Can you work these out from the model? Positions are in its coordinate system, mm. A direction names the side the tool comes from. Give positions to 0.01 mm unless a question says otherwise; leave off trailing zeros. Order: outer loops, then holes, each group sorted by start corner. A loop starts at its lowest first (then second) coordinate and runs counter-clockwise, first axis right, second up. Notation, with made-up numbers: (-12.5, 42.25) - (-4.5, 42.25) arc R23 cw to (-4.5, 62.25) - close; hole circle Ø9 at (43.25, -5.5). An arc over 180 degrees is marked (long way). Answer as a JSON object with one key per item and string values.
```python
from build123d import *

# Parameters (mm, degrees)
SKETCH1_W           = 27.99800038
SKETCH1_H           = 2
BOSS_EXTRUDE1_DEPTH = 10
CUT_EXTRUDE1_DEPTH  = 32
SKETCH4_W           = 27.99800038
SKETCH4_H           = 2
BOSS_EXTRUDE2_DEPTH = 22.81231465
SKETCH5_W           = 4.9
SKETCH5_H           = 2
BOSS_EXTRUDE3_DEPTH = 27.99800038


with BuildPart() as part:
    # Sketch1 → Boss-Extrude1 (new body)
    with BuildSketch(Plane(origin=(0, 0, 0), x_dir=(1, 0, 0), z_dir=(0, 1, 0))):
        with Locations((13.99900019, 1)):
            Rectangle(SKETCH1_W, SKETCH1_H)
    extrude(amount=BOSS_EXTRUDE1_DEPTH)

    # Sketch3 → Cut-Extrude1 (cut)
    with BuildSketch(Plane(origin=(27.99800038, 0, 0), x_dir=(0, 0, -1), z_dir=(1, 0, 0))):
        Polygon((1, 8.25), (2, 8.25), (2, 0), (0, 0), (0, 1), align=None)
    extrude(amount=-CUT_EXTRUDE1_DEPTH, mode=Mode.SUBTRACT)

    # Sketch4 → Boss-Extrude2 (add)
    with BuildSketch(Plane(origin=(0, 10, 0), x_dir=(1, 0, 0), z_dir=(0, 1, 0))):
        with Locations((13.99900019, 1)):
            Rectangle(SKETCH4_W, SKETCH4_H)
    extrude(amount=BOSS_EXTRUDE2_DEPTH)

    # Sketch5 → Boss-Extrude3 (add)
    with BuildSketch(Plane(origin=(27.99800038, 0, 0), x_dir=(0, 0, -1), z_dir=(1, 0, 0))):
        with Locations((2.45, 31.81231465)):
            Rectangle(SKETCH5_W, SKETCH5_H)
        with Locations((2.45, 25.81231465)):
            Rectangle(SKETCH5_W, SKETCH5_H)
    extrude(amount=-BOSS_EXTRUDE3_DEPTH)


solid = part.part
```
Q1. Which directions (+Z, -Z, +X, -X, +Y, -Y) give clear straight access to the entire face, cutting with the end or side of a thin tool? Please do faces 1 (the face through (14, 17, 0)), 2 (the face through (14, 30.812, -3)), 3 (the face through (14.2, 8.25, -1.5)).
Recorded:
{"face 1": "+Z, +X, -X, +Y, -Y", "face 2": "-Z, +X, -X", "face 3": "-Z, +X, -X, -Y"}
Q2. We'd pull the mould along Y, two halves only. Please class faces 4 (the face through (14, 32.812, -2)), 5 (the face through (27.998, 20, -1)), 6 (the face through (14, 24.812, -3)), 7 (the face through (14, 29, -2)): released by +Y, released by -Y, zero draft, split by the parting line, or undercut.
Recorded:
{"face 4": "released by +Y", "face 5": "zero draft", "face 6": "released by -Y", "face 7": "undercut"}
Q3. If we section it at B-B, the plane x = 19: Please give me the cut outline in (y, z).
Recorded:
{"outline": "(1, 0) - (8.25, -1) - (8.25, -2) - (24.81, -2) - (24.81, -4.9) - (26.81, -4.9) - (26.81, -2) - (30.81, -2) - (30.81, -4.9) - (32.81, -4.9) - (32.81, 0) - close"}
Q4. If we section it at C-C, the plane y = 17.5: Please give me the cut outline in (x, z), then the cut area to 3 significant figures.
Recorded:
{"outline": "(0, -2) - (28, -2) - (28, 0) - (0, 0) - close", "area": "56.0 mm^2"}
Q5. If we section it at D-D, the plane z = -0.45: Please give me the cut outline in (x, y).
Recorded:
{"outline": "(0, 4.26) - (28, 4.26) - (28, 32.81) - (0, 32.81) - close"}
Q6. If we section it at A-A, the plane z = -2.4: Please give me the cut outline in (x, y).
Recorded:
{"outline": "(0, 24.81) - (28, 24.81) - (28, 26.81) - (0, 26.81) - close; (0, 30.81) - (28, 30.81) - (28, 32.81) - (0, 32.81) - close"}
Q7. I'm going to push flat-ended pins straight in: pin 1 Ø0.9 at (x, z) = (9, -2.5) entering from -Y; pin 2 Ø5 at (x, y) = (11, 19.5) entering from -Z; pin 3 Ø0.5 at (x, z) = (11, -1.5) entering from -Y. Where does each tip first touch, or does it pass through?
Recorded:
{"pin 1": "stops at y = 24.81", "pin 2": "stops at z = -2", "pin 3": "stops at y = 8.25"}
Q8. I need wall thicknesses on L1, parallel to Y at x = 26, z = -4.6; L2, parallel to Z at x = 10.25, y = 18; L3, parallel to Y at x = 9.5, z = -1.55. Which ranges of each line are inside material? Lowest first, please.
Recorded:
{"L1": "y = 24.81 to 26.81, 30.81 to 32.81", "L2": "z = -2 to 0", "L3": "y = 8.25 to 32.81"}
